Can you work these out from the model? Positions are in its coordinate system, mm. Face numbers are marked on the shaded views. Give positions to 0.01 mm unless a question says otherwise; leave off trailing zeros. Write each loop counter-clockwise with the first axis right and the second up, starting at its lowest first coordinate (ties: lowest second). Pieces come first, ordered by that corner, then holes. Notation, with made-up numbers: (-8, 47.25) -> (35, 47.25) arc R27 ccw to (35, 67.25) -> close; hole circle Ø6 at (-23.75, -17). An arc over 180 degrees is marked (long way). Answer as CSV lines item,"result". Start each with the question number.
1. I need wall thicknesses on line 1 (Z direction, x = 6.75, y = 11.7); line 2 (Z direction, x = 19.5, y = -5.5); line 3 (Y direction, x = 22, z = 109). Which ranges of each line are inside material? Lowest first, please. Write a range as [from, to].
2. If we mould it in two halves opening along Y, with no side actions, what happens to the marked faces 1, 2 and 3? For each: pulls with the +Y half, pulls with the -Y half, needs draft (parallel to the pull), parting line crosses it, or undercut.
3. I'm going to push flat-ended pins straight in: P1, Ø6, axis at x = 17.5, y = -9.5, coming from the +Z side; P2, Ø8, axis at x = 30, y = -3.5, coming from the -Z side. Where does each tip first touch, or does it pass through?
4. If we section it at A-A on x = 32.5: Write out the boundary of the cut face in (y, z).
5. If we section it at B-B on y = 2.25: Write out the boundary of the cut face in (x, z), plus the area to 3 significant figures.
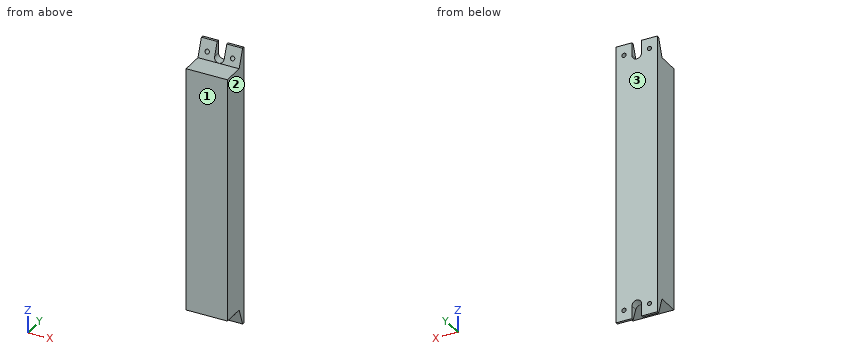
```python
from build123d import *

# Parameters (mm, degrees)
RESSALTO_EXTRUS_O1_DEPTH = 35.2
ESBO_O2_R                = 1.8
CORTE_EXTRUS_O1_DEPTH    = 35.2


with BuildPart() as part:
    # Esboço1 → Ressalto-extrusão1 (new body)
    with BuildSketch(Plane(origin=(0, 0, 0), x_dir=(0, 0, -1), z_dir=(1, 0, 0))):
        Polygon((-105, 13.15), (-120, 13.15), (-120, 11.15), (-105, 5.65), (-105, -13.15), (105, -13.15), (105, 5.65), (120, 11.15), (120, 13.15), (105, 13.15), align=None)
    extrude(amount=RESSALTO_EXTRUS_O1_DEPTH)

    # Esboço2 → Corte-extrusão1 (cut)
    with BuildSketch(Plane.XZ.offset(13.15)):
        with Locations((6.75, 111)):
            Circle(ESBO_O2_R)
        with Locations((28.45, 111)):
            Circle(ESBO_O2_R)
        with Locations((28.45, -111)):
            Circle(ESBO_O2_R)
        with Locations((6.75, -111)):
            Circle(ESBO_O2_R)
        with BuildLine():
            Line((13.5, 109.1), (13.5, 120))
            Line((13.5, 120), (21.7, 120))
            Line((21.7, 120), (21.7, 109.1))
            ThreePointArc((21.7, 109.1), (17.6, 105), (13.5, 109.1))
        make_face()
        with BuildLine():
            Line((13.5, -120), (21.7, -120))
            Line((21.7, -120), (21.7, -109.1))
            ThreePointArc((21.7, -109.1), (17.6, -105), (13.5, -109.1))
            Line((13.5, -109.1), (13.5, -120))
        make_face()
    extrude(amount=-CORTE_EXTRUS_O1_DEPTH, mode=Mode.SUBTRACT)


solid = part.part
```
Computed values:
1,line 1,"z = [-120, -112.8], [-109.2, 109.2], [112.8, 120]"
1,line 2,"z = [-105, 105]"
1,line 3,"y = [7.12, 13.15]"
2,face 1,"pulls with the -Y half"
2,face 2,"needs draft"
2,face 3,"pulls with the +Y half"
3,P1,"stops at z = 105"
3,P2,"stops at z = -105"
4,outline,"(-13.15, -105) -> (5.65, -105) -> (11.15, -120) -> (13.15, -120) -> (13.15, 120) -> (11.15, 120) -> (5.65, 105) -> (-13.15, 105) -> close"
5,outline,"(0, -105) -> (35.2, -105) -> (35.2, 105) -> (0, 105) -> close"
5,area,"7,390 mm2"
